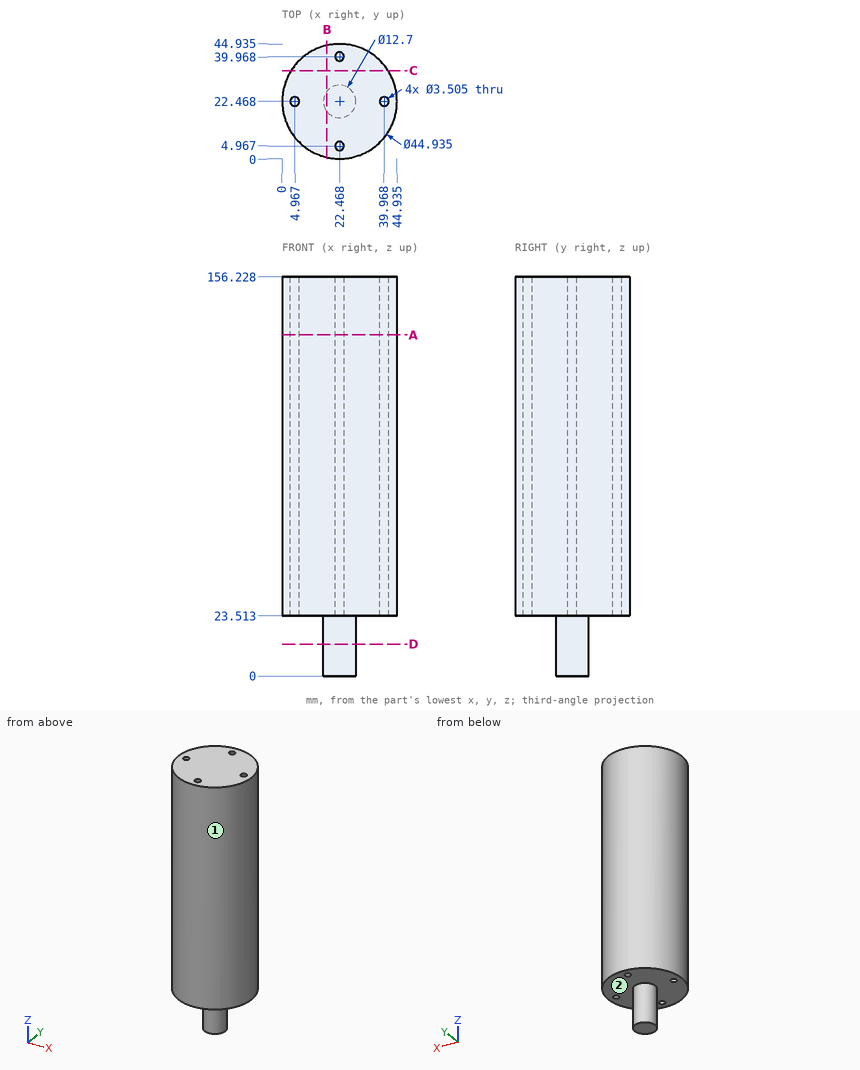
The figure shows three views and two pictorial views of one solid part (mm, origin at its lowest corner). Answer the questions. A direction names the side the tool comes from. Round coordinates to 2 decimals unless told otherwise and drop trailing zeros. Loops run counter-clockwise (first coordinate to the right, second up) from the corner with the lowest first, then second, coordinate; pieces in that order, holes last. Notation, with made-up numbers: (53.25, 67) -> (88.25, 67) arc R19 ccw to (88.25, 99) -> close; hole circle Ø9 at (75.25, 7.25). An arc over 180 degrees is marked (long way). Use one line per item in the form item = value.
(1) Straight lines are drawn through the part: line 1 (X direction, y = 21.5, z = 30) (1 decimal); line 2 (Z direction, x = 22.5, y = 7); line 3 (X direction, y = 39.5, z = 66) (1 decimal). For each, find the intervals that lie inside material, in ascending order.
Answer list:
line_1 = 0 to 3.5, 6.4 to 38.5, 41.4 to 44.9
line_2 = 23.51 to 156.23
line_3 = 7.8 to 20.8, 24.2 to 37.1
(2) Find section A-A on z = 133.5. Give the vertices of the cut face in (x, y) (1 decimal).
Answer list:
outline = circle Ø44.9 at (22.5, 22.5); hole circle Ø3.5 at (5, 22.5); hole circle Ø3.5 at (22.5, 5); hole circle Ø3.5 at (22.5, 40); hole circle Ø3.5 at (40, 22.5)
(3) Find section C-C on y = 34.5. Give the vertices of the cut face in (x, z), then the cut area to 3 significant figures.
Answer list:
outline = (3.49, 23.51) -> (41.44, 23.51) -> (41.44, 156.23) -> (3.49, 156.23) -> close
area = 5,040 mm2
(4) Find section B-B on x = 17.5. Give the vertices of the cut face in (y, z), then the cut area to 3 significant figures.
Answer list:
outline = (0.56, 23.51) -> (18.51, 23.51) -> (18.51, 0) -> (26.42, 0) -> (26.42, 23.51) -> (44.38, 23.51) -> (44.38, 156.23) -> (0.56, 156.23) -> close
area = 6,000 mm2
(5) Flat-ended cylindrical pins translate along their axes: P1, Ø4, axis at x = 22.47, y = 4.97, coming from the -Z side; P2, Ø3, axis at x = 22.47, y = 39.97, coming from the -Z side; P3, Ø12, axis at x = 6, z = 44.5, coming from the -Y side; P4, Ø2, axis at y = 11, z = 71, coming from the +X side. Find the tip coordinate at first contact, or state that the pin passes through.
Answer list:
P1 = 23.51
P2 = through
P3 = 2.59
P4 = 42.35
(6) Find section D-D on z = 12.5. Give the vertices of the cut face in (x, y), then the cut area to 3 significant figures.
Answer list:
outline = circle Ø12.7 at (22.47, 22.47)
area = 127 mm2
(7) A tool of negligible diameter and unlimited length cuts with its end or side. For the marked faces 1 and 2, from which of +Z, -Z, +X, -X, +Y, -Y can it reach the whole face along a straight path? Write none if from no direction.
Answer list:
face_1 = +Z, -Z
face_2 = -Z
